```python
from build123d import *

# Parameters (mm, degrees)
SKETCH1_R             = 3.6
SKETCH1_R_2           = 2.55
BOSS_EXTRUDE1_DEPTH   = 6
M5X0_8_TAPPED_HOLE1_D = 4.2
SKETCH2_R             = 6
SKETCH2_R_2           = 4.5
CUT_EXTRUDE1_DEPTH    = 1.5


with BuildPart() as part:
    # Sketch1 → Boss-Extrude1 (new body)
    with BuildSketch(Plane(origin=(0, 0, 0), x_dir=(1, 0, 0), z_dir=(0, 1, 0))):
        with BuildLine():
            Line((33.94, -38.575), (-33.94, -38.575))
            ThreePointArc((-33.94, -38.575), (-37.217439931, -37.217439931), (-38.575, -33.94))
            Line((-38.575, -33.94), (-38.575, 33.94))
            ThreePointArc((-38.575, 33.94), (-37.217439931, 37.217439931), (-33.94, 38.575))
            Line((-33.94, 38.575), (33.94, 38.575))
            ThreePointArc((33.94, 38.575), (37.217439931, 37.217439931), (38.575, 33.94))
            Line((38.575, 33.94), (38.575, -33.94))
            ThreePointArc((38.575, -33.94), (37.217439931, -37.217439931), (33.94, -38.575))
        make_face()
        with Locations((-30, 14.25)):
            Circle(SKETCH1_R, mode=Mode.SUBTRACT)
        with Locations((-20, 10)):
            Circle(SKETCH1_R_2, mode=Mode.SUBTRACT)
        with Locations((0, 20)):
            Circle(SKETCH1_R_2, mode=Mode.SUBTRACT)
        with Locations((0, 10)):
            Circle(SKETCH1_R_2, mode=Mode.SUBTRACT)
        with Locations((-10, 10)):
            Circle(SKETCH1_R_2, mode=Mode.SUBTRACT)
        with Locations((-30, 30)):
            Circle(SKETCH1_R_2, mode=Mode.SUBTRACT)
        with Locations((-30, 0)):
            Circle(SKETCH1_R_2, mode=Mode.SUBTRACT)
        with Locations((30, 30)):
            Circle(SKETCH1_R_2, mode=Mode.SUBTRACT)
        with Locations((30, 14.25)):
            Circle(SKETCH1_R, mode=Mode.SUBTRACT)
        with Locations((30, 0)):
            Circle(SKETCH1_R_2, mode=Mode.SUBTRACT)
        with Locations((20, 10)):
            Circle(SKETCH1_R_2, mode=Mode.SUBTRACT)
        with Locations((20, -10)):
            Circle(SKETCH1_R_2, mode=Mode.SUBTRACT)
        with Locations((-30, -30)):
            Circle(SKETCH1_R_2, mode=Mode.SUBTRACT)
        with Locations((30, -30)):
            Circle(SKETCH1_R_2, mode=Mode.SUBTRACT)
        with Locations((-20, -10)):
            Circle(SKETCH1_R_2, mode=Mode.SUBTRACT)
        with Locations((0, -20)):
            Circle(SKETCH1_R_2, mode=Mode.SUBTRACT)
        with Locations((0, -10)):
            Circle(SKETCH1_R_2, mode=Mode.SUBTRACT)
        with Locations((-10, -10)):
            Circle(SKETCH1_R_2, mode=Mode.SUBTRACT)
        with Locations((10, 0)):
            Circle(SKETCH1_R_2, mode=Mode.SUBTRACT)
        with Locations((30, -14.25)):
            Circle(SKETCH1_R_2, mode=Mode.SUBTRACT)
        with Locations((-30, -14.25)):
            Circle(SKETCH1_R_2, mode=Mode.SUBTRACT)
        with BuildLine():
            Line((0, -2.55), (-10, -2.55))
            ThreePointArc((-10, -2.55), (-12.55, 0), (-10, 2.55))
            Line((-10, 2.55), (0, 2.55))
            ThreePointArc((0, 2.55), (2.55, 0), (0, -2.55))
        make_face(mode=Mode.SUBTRACT)
    extrude(amount=BOSS_EXTRUDE1_DEPTH)

    # M5x0.8 Tapped Hole1 (through all)
    with Locations(Plane(origin=(0, 6, 0), x_dir=(1, 0, 0), z_dir=(0, 1, 0))):
        with Locations((-20, 20), (-10, 30), (10, 30), (20, 20), (20, -20), (10, -30), (-10, -30), (-20, -20)):
            Hole(M5X0_8_TAPPED_HOLE1_D / 2)

    # Sketch2 → Cut-Extrude1 (cut)
    with BuildSketch(Plane(origin=(0, 6, 0), x_dir=(1, 0, 0), z_dir=(0, 1, 0))):
        with Locations((-30, 14.25)):
            Circle(SKETCH2_R)
        with Locations((30, 14.25)):
            Circle(SKETCH2_R)
        with Locations((30, -14.25)):
            Circle(SKETCH2_R_2)
        with Locations((-30, -14.25)):
            Circle(SKETCH2_R_2)
        with BuildLine():
            Line((10.03, -14.95), (-10.03, -14.95))
            ThreePointArc((-10.03, -14.95), (-13.508965363, -13.508965363), (-14.95, -10.03))
            Line((-14.95, -10.03), (-14.95, 10.03))
            ThreePointArc((-14.95, 10.03), (-13.508965363, 13.508965363), (-10.03, 14.95))
            Line((-10.03, 14.95), (10.03, 14.95))
            ThreePointArc((10.03, 14.95), (13.508965363, 13.508965363), (14.95, 10.03))
            Line((14.95, 10.03), (14.95, -10.03))
            ThreePointArc((14.95, -10.03), (13.508965363, -13.508965363), (10.03, -14.95))
        make_face()
    extrude(amount=-CUT_EXTRUDE1_DEPTH, mode=Mode.SUBTRACT)


solid = part.part
```
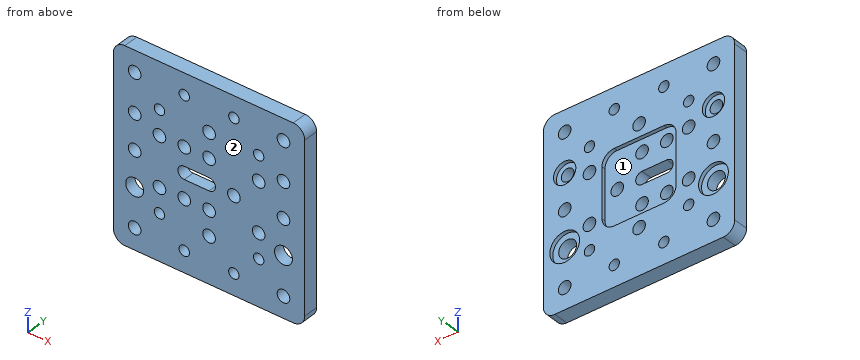
Geometry check sheet. Reference: the model listing, model coordinates, mm. Face numbers are marked on the shaded views. A direction names the side the tool comes from. Coordinates: 2 decimals unless noted, no trailing zeros. Order: outer loops, then holes, each group sorted by start corner. A loop starts at its lowest first (then second) coordinate and runs counter-clockwise, first axis right, second up. Notation, with made-up numbers: M -7,-12.5 L 43,-12.5 A7 ccw 43,-8.5 Z; hole C -25,16 d3. An arc over 180 degrees is marked long. Answer as a JSON object with one key per item and string values.
Q1. Cross-section at A-A on x = -20. Record the cut outline in (y, z) (3 decimals), and give its area (3 significant figures).
Results are:
{"outline": "M 0,-38.575 L 6,-38.575 L 6,-22.1 L 0,-22.1 Z; M 0,-17.9 L 6,-17.9 L 6,-12.55 L 0,-12.55 Z; M 0,-7.45 L 6,-7.45 L 6,7.45 L 0,7.45 Z; M 0,12.55 L 6,12.55 L 6,17.9 L 0,17.9 Z; M 0,22.1 L 6,22.1 L 6,38.575 L 0,38.575 Z", "area": "351 mm²"}
Q2. Depth check by flat-ended pin: pin 1 Ø3.5 at (x, z) = (20, -20) entering from +Y; pin 2 Ø6.5 at (x, z) = (30, 14.25) entering from +Y. Enter the tip coordinate at first touch or a pass-through.
Results are:
{"pin 1": "passes through", "pin 2": "stops at y = 4.5"}
Q3. Cross-section at B-B on z = 20. Record the cut outline in (x, y) (3 decimals), and give its area (3 significant figures).
Results are:
{"outline": "M -38.575,0 L -22.1,0 L -22.1,6 L -38.575,6 Z; M -17.9,0 L -2.55,0 L -2.55,6 L -17.9,6 Z; M 2.55,0 L 17.9,0 L 17.9,6 L 2.55,6 Z; M 22.1,0 L 38.575,0 L 38.575,6 L 22.1,6 Z", "area": "382 mm²"}
Q4. Cross-section at C-C on x = -30. Give the number of separate pieces and of enclosed holes in the cut face, and give its area (3 significant figures).
Results are:
{"separate pieces": "6", "enclosed holes": "0", "area": "284 mm²"}
Q5. Tool access check on the marked faces 1 and 2. Record the directions out of +Z, -Z, +X, -X, +Y, -Y that give a thin tool (end or side, any length) a straight path to the whole face; none if there is none.
Results are:
{"face 1": "+Y", "face 2": "+Z, -Z, +X, -X, -Y"}
Q6. Cross-section at D-D on z = -5. Record the cut outline in (x, y) (3 decimals).
Results are:
{"outline": "M -38.575,0 L 38.575,0 L 38.575,6 L 14.95,6 L 14.95,4.5 L -14.95,4.5 L -14.95,6 L -38.575,6 Z"}
Q7. Scan lines: line 1 (X direction, y = 1.7, z = 14.25) (3 decimals); line 2 (X direction, y = 3.4, z = -10) (3 decimals); line 3 (X direction, y = 3.3, z = 30) (3 decimals). Record each from-to range of solid material in increasing order.
Results are:
{"line 1": "x = -38.575 to -32.55, -27.45 to 27.45, 32.55 to 38.575", "line 2": "x = -38.575 to -22.55, -17.45 to -12.55, -7.45 to -2.55, 2.55 to 17.45, 22.55 to 38.575", "line 3": "x = -38.575 to -32.55, -27.45 to -12.1, -7.9 to 7.9, 12.1 to 27.45, 32.55 to 38.575"}
